Verification items for the finished model (mm, model axes). A direction names the side the tool comes from. Give positions to 0.01 mm unless a question says otherwise; leave off trailing zeros. Order: outer loops, then holes, each group sorted by start corner. A loop starts at its lowest first (then second) coordinate and runs counter-clockwise, first axis right, second up. Notation, with made-up numbers: (7.5, 88.25) - (30.5, 88.25) arc R23 ccw to (30.5, 100.25) - close; hole circle Ø6 at (4.25, -2.75). An arc over 180 degrees is marked (long way). Answer as a JSON object with one key per item and string values. Group by question number.
(1) Section check A-A (y = 266). Record the boundary of the cut face in (x, z).
(2) Thickness scan on line 1 (Y direction, x = -153, z = 5); line 2 (Y direction, x = -285, z = 6.75); line 3 (Y direction, x = -279.5, z = 6.5). Record the ranges inside material, lowest first.
(3) Depth check by flat-ended pin: pin 1 Ø3 at (x, z) = (-280.5, 3) entering from +Y; pin 2 Ø5 at (y, z) = (68, 3.5) entering from +X; pin 3 Ø2 at (y, z) = (312, 3.5) entering from +X. Enter the tip coordinate at first touch or a pass-through.
(4) Access from +Z, -Z, +X, -X, +Y, -Y to the whole of each face (thin tool, end or side, straight path). Record for faces 1 (the face through (0, 268, 5)), 2 (the face through (10, 204, 5)), 3 (the face through (-262, 418, 5)).
(5) Mould release check, pull along X, two halves, no side actions. Record for faces 4 (the face through (-120, 305, 5)), 5 (the face through (-24.791, 129.393, 4.816)), 6 (the face through (-305, 150, 5)): +X half, -X half, draft (parallel to the pull), parting line (faces both ways), or undercut.
(6) Section check C-C (y = 20). Record the boundary of the cut face in (x, z), then the cut area to 3 significant figures.
(7) Section check D-D (x = -153). Record the boundary of the cut face in (y, z).
(8) Section check B-B (x = -203). Record the boundary of the cut face in (y, z), then the cut area to 3 significant figures.
Autodesk Inventor part; units mm, degrees
ref_plane "YZ Plane" through (0, 0, 0) normal (1, 0, 0) x (0, 1, 0)
ref_plane "XZ Plane" through (0, 0, 0) normal (0, 1, 0) x (-1, 0, 0)
ref_plane "XY Plane" through (0, 0, 0) normal (0, 0, 1) x (1, 0, 0)
sketch "Sketch1" plane through (0, 0, 0) normal (0, 0, 1) x (1, 0, 0)
  line L0 (0, 0) -> (-305, 0)
  line L1 (-305, 0) -> (-305, 305)
  line L2 (-305, 305) -> (-262, 305)
  line L3 (-262, 305) -> (-262, 535)
  line L4 (-262, 535) -> (-237, 535)
  line L5 (-237, 535) -> (-237, 305)
  line L6 (-237, 305) -> (0, 305)
  line L7 (0, 305) -> (0, 229)
  line L8 (0, 229) -> (20, 229)
  line L9 (20, 229) -> (20, 204)
  line L10 (20, 204) -> (0, 204)
  line L11 (0, 204) -> (0, 0)
  dimension "d0" = 305
  dimension "d1" = 305
  dimension "d4" = 230
  dimension "d5" = 25
  dimension "d6" = 230
  dimension "d7" = 76
  dimension "d8" = 20
  dimension "d9" = 25
  dimension "d10" = 43
extrude "Extrusion1" add sketch "Sketch1" along normal blind 9.5
sketch "Sketch2" plane through (0, 0, 9.5) normal (0, 0, 1) x (1, 0, 0)
  circle A0 centre (-20, 20) radius 6.5
  circle A1 centre (-20, 125) radius 6.5
  circle A2 centre (-285, 20) radius 6.5
  circle A3 centre (-285, 125) radius 6.5
  circle A4 centre (-153, 166) radius 6.25
  circle A5 centre (-153, 216) radius 25.5
  circle A6 centre (9, 216) radius 4
  line L0 (-305, 0) -> (0, 0)
  circle A7 centre (-103, 216) radius 6.25
  circle A8 centre (-153, 266) radius 6.25
  circle A9 centre (-203, 216) radius 6.25
  dimension "d13" = 13
  dimension "d14" = 13
  dimension "d15" = 13
  dimension "d16" = 13
  dimension "d18" = 12.5
  dimension "d21" = 8
  dimension "d22" = 20
  dimension "d23" = 20
  dimension "d24" = 20
  dimension "d25" = 20
  dimension "d26" = 125
  dimension "d27" = 20
  dimension "d28" = 20
  dimension "d29" = 125
  dimension "d30" = 216
  dimension "d31" = 216
  dimension "d32" = 166
  dimension "d35" = 360
  dimension "d37" = 51
  dimension "d38" = 103
  dimension "d39" = 162
  dimension "d40" = 162
extrude "Extrusion2" cut sketch "Sketch2" against normal through all contours A0 | A1 | A2 | A3 | A4 | A6 | A7 | A8 | A9
sketch "Sketch3" plane through (0, 0, 9.5) normal (0, 0, 1) x (1, 0, 0)
  circle A0 centre (-203, 216) radius 6.25
  circle A1 centre (-103, 216) radius 6.25
  circle A2 centre (-153, 216) radius 25
  circle A3 centre (-285, 125) radius 6.5
  circle A4 centre (-20, 125) radius 6.5
  circle A5 centre (-153, 125) radius 12.7
  point P0 (0, 0)
  dimension "d43" = 50
  dimension "d44" = 216
  dimension "d45" = 153
  dimension "d46" = 25.4
  dimension "d47" = 125
  dimension "d48" = 153
extrude "Extrusion3" cut sketch "Sketch3" against normal through all contours A2 | A5
properties part number "HubPlate"
Solutions:
{
 "1": {"outline": "(-305, 0) - (-159.25, 0) - (-159.25, 9.5) - (-305, 9.5) - close; (-146.75, 0) - (0, 0) - (0, 9.5) - (-146.75, 9.5) - close"},
 "2": {"line 1": "y = 0 to 112.3, 137.7 to 159.75, 172.25 to 191, 241 to 259.75, 272.25 to 305", "line 2": "y = 0 to 13.5, 26.5 to 118.5, 131.5 to 305", "line 3": "y = 0 to 16.54, 23.46 to 121.54, 128.46 to 305"},
 "3": {"pin 1": "stops at y = 305", "pin 2": "stops at x = 0", "pin 3": "stops at x = -237"},
 "4": {"face 1": "+Z, -Z, +X, +Y", "face 2": "+Z, -Z, +X, -Y", "face 3": "+Z, -Z, -X, +Y"},
 "5": {"face 4": "draft", "face 5": "undercut", "face 6": "-X half"},
 "6": {"outline": "(-305, 0) - (-291.5, 0) - (-291.5, 9.5) - (-305, 9.5) - close; (-278.5, 0) - (-26.5, 0) - (-26.5, 9.5) - (-278.5, 9.5) - close; (-13.5, 0) - (0, 0) - (0, 9.5) - (-13.5, 9.5) - close", "area": "2,650 mm2"},
 "7": {"outline": "(0, 0) - (112.3, 0) - (112.3, 9.5) - (0, 9.5) - close; (137.7, 0) - (159.75, 0) - (159.75, 9.5) - (137.7, 9.5) - close; (172.25, 0) - (191, 0) - (191, 9.5) - (172.25, 9.5) - close; (241, 0) - (259.75, 0) - (259.75, 9.5) - (241, 9.5) - close; (272.25, 0) - (305, 0) - (305, 9.5) - (272.25, 9.5) - close"},
 "8": {"outline": "(0, 0) - (209.75, 0) - (209.75, 9.5) - (0, 9.5) - close; (222.25, 0) - (305, 0) - (305, 9.5) - (222.25, 9.5) - close", "area": "2,780 mm2"}
}
